Verification items for this drawing (mm, ordinates from the low corner). A direction names the side the tool comes from. Round coordinates to 2 decimals unless told otherwise and drop trailing zeros. Loops run counter-clockwise (first coordinate to the right, second up) from the corner with the lowest first, then second, coordinate; pieces in that order, holes last. Notation, with made-up numbers: M -14,-13.5 L 30,-13.5 A10 ccw 30,-9.5 Z; hole C 24.25,55 d5. An arc over 180 degrees is marked long. One line per item, written item: value.
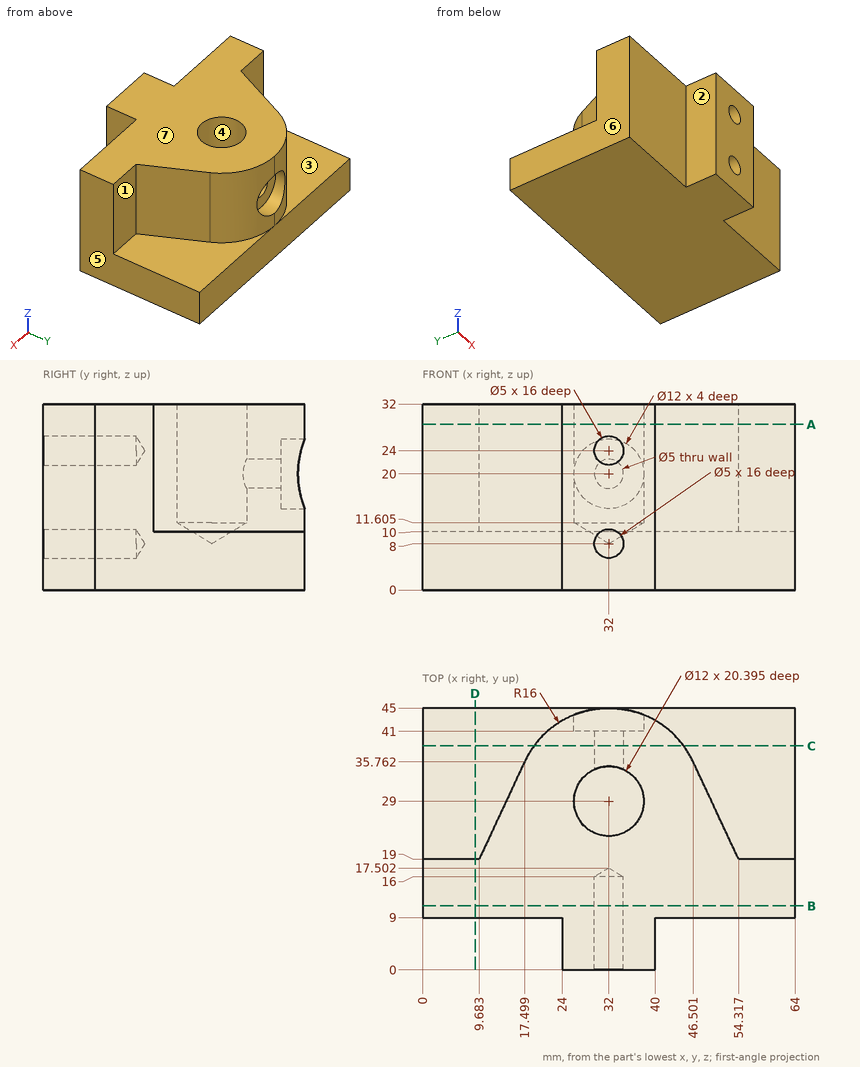
(1) Sectioned sample at A-A on z = 28.5. Enter the section's corners in (x, y), and give its area (3 significant figures).
Completed:
outline: M 0,9 L 24,9 L 24,0 L 40,0 L 40,9 L 64,9 L 64,19 L 54.32,19 L 46.5,35.76 A16 ccw 17.5,35.76 L 9.68,19 L 0,19 Z; hole C 32,29 d12
area: 1,480 mm^2
(2) Thickness scan on L1, parallel to Z at x = 32, y = 9; L2, parallel to Z at x = 32, y = 42.65; L3, parallel to Z at x = 52.5, y = 36. Record the ranges inside material, lowest first. Write a range as from..to.
Completed:
L1: z = 0..5.5, 10.5..21.5, 26.5..32
L2: z = 0..14, 26..32
L3: z = 0..10
(3) Depth check by flat-ended pin: pin 1 Ø7 at (y, z) = (5, 16.5) entering from +X; pin 2 Ø4 at (y, z) = (30.5, 20) entering from +X; pin 3 Ø7 at (x, z) = (32, 20) entering from +Y. Enter the tip coordinate at first touch or a pass-through.
Completed:
pin 1: stops at x = 40
pin 2: stops at x = 49.89
pin 3: stops at y = 41
(4) Sectioned sample at B-B on y = 11. Enter the section's corners in (x, z).
Completed:
outline: M 0,0 L 64,0 L 64,32 L 0,32 Z; hole C 32,8 d5; hole C 32,24 d5
(5) Tool access check on the marked faces 1, 2 and 3. Record the directions out of +Z, -Z, +X, -X, +Y, -Y that give a thin tool (end or side, any length) a straight path to the whole face; none if there is none.
Completed:
face 1: +Z, +X, +Y
face 2: +Z, -Z, -X, -Y
face 3: +Z, -X, +Y
(6) Sectioned sample at D-D on x = 9. Enter the section's corners in (y, z), and give its area (3 significant figures).
Completed:
outline: M 9,0 L 45,0 L 45,10 L 19,10 L 19,32 L 9,32 Z
area: 580 mm^2
(7) Mould release check, pull along X, two halves, no side actions. Record for the marked faces 4, 5, 6 and 7: +X half, -X half, draft (parallel to the pull), parting line (faces both ways), or undercut.
Completed:
face 4: undercut
face 5: +X half
face 6: -X half
face 7: draft
(8) Sectioned sample at C-C on y = 38.5. Enter the section's corners in (x, z).
Completed:
outline: M 0,0 L 64,0 L 64,10 L 44.87,10 L 44.87,32 L 19.13,32 L 19.13,10 L 0,10 Z; hole C 32,20 d5
